Input: part model. Units: mm. Frame: model coordinates. A direction names the side the tool comes from. Give positions to 0.01 mm unless a question says otherwise; leave off trailing zeros. Loops run counter-clockwise (first coordinate to the right, second up) from the corner with the lowest first, then second, coordinate; pieces in that order, holes last.
from build123d import *

# Parameters (mm, degrees)
SKETCH_1_W           = 50
SKETCH_1_H           = 80
EXTRUDE_1_DEPTH      = 80
SKETCH_4_W           = 50
SKETCH_4_H           = 160
CUT_REVOLVE_2_ANGLE  = 20
SKETCH_5_W           = 100
SKETCH_5_H           = 160
CUT_REVOLVE_4_ANGLE  = 43.2
SKETCH_6_W           = 10
SKETCH_6_H           = 80
SKETCH_6_W_2         = 10.000248079
CUT_EXTRUDE_1_DEPTH  = 80
SKETCH_7_W           = 5.91
SKETCH_7_H           = 80
CUT_EXTRUDE_2_DEPTH  = 50
SHELL_2_T            = 3
SKETCH_8_W           = 19.999751921
SKETCH_8_H           = 70
CUT_EXTRUDE_3_DEPTH  = 3
CUT_EXTRUDE_4_DEPTH  = 3
CUT_EXTRUDE_5_DEPTH  = 3
CUT_EXTRUDE_6_DEPTH  = 3
CUT_EXTRUDE_7_DEPTH  = 3
CUT_EXTRUDE_9_DEPTH  = 3
SKETCH_18_W          = 2
SKETCH_18_H          = 20
EXTRUDE_2_DEPTH      = 10
SKETCH_19_W          = 2
SKETCH_19_H          = 20
EXTRUDE_3_DEPTH      = 10
SKETCH_20_R          = 2
CUT_EXTRUDE_10_DEPTH = 2


with BuildPart() as part:
    # 草图1 → 凸台-拉伸1 (new body)
    with BuildSketch(Plane.XY):
        Rectangle(SKETCH_1_W, SKETCH_1_H)
    extrude(amount=EXTRUDE_1_DEPTH)

    # 草图4 → 切除-旋转2 (revolve, cut)
    with BuildSketch(Plane.XY.offset(80)):
        with Locations((0, -40)):
            Rectangle(SKETCH_4_W, SKETCH_4_H)
    revolve(axis=Axis((-25, 40, 80), (1, 0, 0)), revolution_arc=CUT_REVOLVE_2_ANGLE, mode=Mode.SUBTRACT)

    # 草图5 → 切除-旋转4 (revolve, cut)
    with BuildSketch(Plane(origin=(0, -21.03239325, 57.786025531), x_dir=(1, 0, 0), z_dir=(0, -0.34202014332566943, 0.9396926207859082))):
        with Locations((25, -15.050683703)):
            Rectangle(SKETCH_5_W, SKETCH_5_H)
    revolve(axis=Axis((-25, 40, 80), (0, 0.9396926207859082, 0.3420201433256695)), revolution_arc=CUT_REVOLVE_4_ANGLE, mode=Mode.SUBTRACT)

    # 草图6 → 切除-拉伸1 (cut)
    with BuildSketch(Plane(origin=(0, 0, 0), x_dir=(-1, 0, 0), z_dir=(0, 0, -1))):
        with Locations((-20, 0)):
            Rectangle(SKETCH_6_W, SKETCH_6_H)
        with Locations((19.99987596, 0)):
            Rectangle(SKETCH_6_W_2, SKETCH_6_H)
    extrude(amount=-CUT_EXTRUDE_1_DEPTH, mode=Mode.SUBTRACT)

    # 草图7 → 切除-拉伸2 (cut)
    with BuildSketch(Plane(origin=(15, 0, 0), x_dir=(0, 0, -1), z_dir=(1, 0, 0))):
        with Locations((-2.955, 0)):
            Rectangle(SKETCH_7_W, SKETCH_7_H)
    extrude(amount=-CUT_EXTRUDE_2_DEPTH, mode=Mode.SUBTRACT)

    # 抽壳2 (no face opened: a closed hollow body)
    add(offset(amount=-SHELL_2_T, mode=Mode.PRIVATE), mode=Mode.SUBTRACT)

    # 草图8 → 切除-拉伸3 (cut)
    with BuildSketch(Plane(origin=(0, 0, 5.91), x_dir=(-1, 0, 0), z_dir=(0, 0, -1))):
        with Locations((-0.000124039, 0)):
            Rectangle(SKETCH_8_W, SKETCH_8_H)
    extrude(amount=-CUT_EXTRUDE_3_DEPTH, mode=Mode.SUBTRACT)

    # 草图9 → 切除-拉伸4 (cut)
    with BuildSketch(Plane(origin=(0, 40, 0), x_dir=(1, 0, 0), z_dir=(0, 1, 0))):
        Polygon((12, -8.91), (-11.999751921, -8.91), (-11.999751921, -62.767250828), (12, -38.783592046), align=None)
    extrude(amount=-CUT_EXTRUDE_4_DEPTH, mode=Mode.SUBTRACT)

    # 草图10 → 切除-拉伸5 (cut)
    with BuildSketch(Plane.XZ.offset(40)):
        Polygon((12.756480566, 8.91), (-11.999751921, 8.91), (-11.999751921, 33.649632087), align=None)
    extrude(amount=-CUT_EXTRUDE_5_DEPTH, mode=Mode.SUBTRACT)

    # 草图11 → 切除-拉伸6 (cut)
    with BuildSketch(Plane.ZY.offset(14.999751921)):
        Polygon((10.91, -30), (10.91, -5), (48.306908226, -5), (39.207652369, -30), align=None)
        Polygon((10.91, 5), (10.91, 30), (61.045866425, 30), (51.946610569, 5), align=None)
    extrude(amount=-CUT_EXTRUDE_6_DEPTH, mode=Mode.SUBTRACT)

    # 草图15 → 切除-拉伸7 (cut)
    with BuildSketch(Plane(origin=(15, 0, 0), x_dir=(0, 0, -1), z_dir=(1, 0, 0))):
        Polygon((-30.80754043, 30), (-10.91, 30), (-10.91, 15), (-25.347986916, 15), align=None)
        Polygon((-10.91, 5), (-10.91, -20), (-12.867719255, -20), (-21.966975112, 5), align=None)
    extrude(amount=-CUT_EXTRUDE_7_DEPTH, mode=Mode.SUBTRACT)

    # 草图17 → 切除-拉伸9 (cut)
    with BuildSketch(Plane(origin=(18.971510682, -6.909698516, 18.984240647), x_dir=(0.7289686274214102, 0.23412889928290287, -0.6432638640215396), z_dir=(0.6845471059286902, -0.24932195443058733, 0.6850064399723311))):
        Polygon((-39.60181704, 0.417311671), (-12.448122913, -6.348160757), (-12.448122913, 27.257474323), (-39.60181704, 34.022946751), align=None)
    extrude(amount=-CUT_EXTRUDE_9_DEPTH, mode=Mode.SUBTRACT)

    # 草图18 → 凸台-拉伸2 (add)
    with BuildSketch(Plane(origin=(15, 0, 0), x_dir=(0, 0, -1), z_dir=(1, 0, 0))):
        with Locations((-6.91, -30)):
            Rectangle(SKETCH_18_W, SKETCH_18_H)
        with Locations((-6.91, 30)):
            Rectangle(SKETCH_18_W, SKETCH_18_H)
    extrude(amount=EXTRUDE_2_DEPTH)

    # 草图19 → 凸台-拉伸3 (add)
    with BuildSketch(Plane.ZY.offset(14.999751921)):
        with Locations((6.91, 30)):
            Rectangle(SKETCH_19_W, SKETCH_19_H)
        with Locations((6.91, -30)):
            Rectangle(SKETCH_19_W, SKETCH_19_H)
    extrude(amount=EXTRUDE_3_DEPTH)

    # 草图20 → 切除-拉伸10 (cut)
    with BuildSketch(Plane(origin=(0, 0, 5.91), x_dir=(-1, 0, 0), z_dir=(0, 0, -1))):
        with BuildLine():
            Line((24.999751921, 32), (19.999751921, 32))
            ThreePointArc((19.999751921, 32), (17.999751921, 30), (19.999751921, 28))
            Line((19.999751921, 28), (24.999751921, 28))
            Line((24.999751921, 28), (24.999751921, 32))
        make_face()
        with BuildLine():
            Line((19.999751921, -32), (24.999751921, -32))
            Line((24.999751921, -32), (24.999751921, -28))
            Line((24.999751921, -28), (19.999751921, -28))
            ThreePointArc((19.999751921, -28), (17.999751921, -30), (19.999751921, -32))
        make_face()
        with Locations(Location((-20, 30, 0), (0, 0, 90))):
            Circle(SKETCH_20_R)
        with Locations(Location((-20, -30, 0), (0, 0, 90))):
            Circle(SKETCH_20_R)
    extrude(amount=-CUT_EXTRUDE_10_DEPTH, mode=Mode.SUBTRACT)


solid = part.part
(1) Cut plane C-C (y = -23). Return the cut outline in (x, z), and give its area (3 significant figures).
Values follow:
outline: (-25, 5.91) - (-10, 5.91) - (-10, 8.91) - (-12, 8.91) - (-12, 10.91) - (-15, 10.91) - (-15, 7.91) - (-25, 7.91) - close; (-15, 41.76) - (-12, 41.76) - (-12, 39.7) - (12, 15.72) - (12, 8.91) - (10, 8.91) - (10, 5.91) - (25, 5.91) - (25, 7.91) - (15, 7.91) - (15, 17.1) - (-15, 47.08) - close
area: 222 mm2
(2) Cut plane A-A (x = 20). Return the cut outline in (y, z).
Values follow:
outline: (-40, 5.91) - (-32, 5.91) - (-32, 7.91) - (-40, 7.91) - close; (-28, 5.91) - (-20, 5.91) - (-20, 7.91) - (-28, 7.91) - close; (20, 5.91) - (28, 5.91) - (28, 7.91) - (20, 7.91) - close; (32, 5.91) - (40, 5.91) - (40, 7.91) - (32, 7.91) - close
(3) Mould query, pull axis X, two halves, no side actions, for faces 4 (the cylindrical face through (-18, 30, 7)), 5 (the flat face through (-10, 0, 7)), 6 (the flat face through (-14, -18, 10.91)). Classes: +X half, -X half, draft (parallel to the pull), parting line (faces both ways), or undercut.
Values follow:
face 4: -X half
face 5: undercut
face 6: draft
(4) Ray query, probe 1 along X at (y, z) = (30, 7.25); probe 2 along X at (y, z) = (33, 29.5); probe 3 along Z at (x, y) = (-11, 23.5). Return the intervals inside material, ascending.
Values follow:
probe 1: x = -18 to -10, 10 to 18, 22 to 25
probe 2: x = -15 to -12, 12 to 15
probe 3: z = 5.91 to 8.91, 55.62 to 60
(5) Cut plane B-B (z = 15.5). Return the cut outline in (x, y).
Values follow:
outline: (-15, -40) - (-12, -40) - (-12, -30) - (-15, -30) - close; (-15, -5) - (-12, -5) - (-12, 5) - (-15, 5) - close; (-15, 30) - (-12, 30) - (-12, 40) - (-15, 40) - close; (6.16, -40) - (10.41, -40) - (15, -27.39) - (15, -12.77) - (12, -12.77) - (12, -23.59) - (7.12, -37) - (6.16, -37) - close; (12, 5) - (15, 5) - (15, 15) - (12, 15) - close; (12, 30) - (15, 30) - (15, 40) - (12, 40) - close
(6) Pin query (flat end, axial travel): pin 1 Ø3 at (x, y) = (-20, 26.5) entering from +Z; pin 2 Ø1.5 at (x, y) = (-14, -15.5) entering from +Z; pin 3 Ø4 at (x, y) = (3.5, -21.5) entering from -Z. Return the tip coordinate at first contact, or that it passes through.
Values follow:
pin 1: stops at z = 7.91
pin 2: stops at z = 49.6
pin 3: stops at z = 22.63
(7) Reachability of faces 1 (the flat face through (-12, 18, 55)), 2 (the flat face through (12, 13, 19)), 3 (the flat face through (-17.7, -30.1, 7.91)) from +Z, -Z, +X, -X, +Y, -Y: full face, straight path, thin tool, end or side. Return the list, or none.
Values follow:
face 1: -X
face 2: +Y
face 3: +Z, -X, +Y, -Y
(8) Cut plane D-D (x = -16.5). Return the cut outline in (y, z), and give its area (3 significant figures).
Values follow:
outline: (-40, 5.91) - (-20, 5.91) - (-20, 7.91) - (-40, 7.91) - close; (20, 5.91) - (40, 5.91) - (40, 7.91) - (20, 7.91) - close
area: 80.0 mm2
